Build history of the part. All positions in model axes, mm. A direction names the side the tool comes from. Round coordinates to 2 decimals unless told otherwise and drop trailing zeros. Write each loop counter-clockwise with the first axis right and the second up, starting at its lowest first coordinate (ties: lowest second). Pieces come first, ordered by that corner, then holes.
from build123d import *

# Parameters (mm, degrees)
EXTRUDE_1_DEPTH          = 26.5
SKETCH_3_R               = 1.5
CUT_EXTRUDE_1_DEPTH      = 53.519044165
SKETCH_3_3_R             = 4
CUT_EXTRUDE_2_DEPTH      = 53.519044165
CUT_EXTRUDE_3_DEPTH      = 53.46189093
CUT_EXTRUDE_3_DEPTH_BACK = 53.46189093
SKETCH_4_R               = 1.5
SKETCH_4_R_2             = 5


with BuildPart() as part:
    # Sketch 2 → Extrude 1 (new body)
    with BuildSketch(Plane.XY):
        with BuildLine():
            Line((0, 1), (0, 34))
            Line((0, 34), (3, 34))
            Line((3, 34), (3, 4))
            ThreePointArc((3, 4), (3.292893219, 3.292893219), (4, 3))
            Line((4, 3), (33, 3))
            Line((33, 3), (33, 0))
            Line((33, 0), (1, 0))
            ThreePointArc((1, 0), (0.292893219, 0.292893219), (0, 1))
        make_face()
    extrude(amount=EXTRUDE_1_DEPTH)

    # Sketch 3 → Cut-Extrude 1 (cut, through all)
    with BuildSketch(Plane(origin=(3, 0, 0), x_dir=(0, 0, -1), z_dir=(1, 0, 0))):
        with BuildLine():
            ThreePointArc((-13.25, 34), (-3.880835149, 30.119164851), (0, 20.75))
            Line((0, 20.75), (0, 34))
            Line((0, 34), (-13.25, 34))
        make_face()
        with BuildLine():
            ThreePointArc((-26.5, 20.75), (-22.619164851, 30.119164851), (-13.25, 34))
            Line((-13.25, 34), (-26.5, 34))
            Line((-26.5, 34), (-26.5, 20.75))
        make_face()
        with Locations(Location((-4.75, 20.75, 0), (0, 0, 90))):
            Circle(SKETCH_3_R)
        with Locations(Location((-21.75, 20.75, 0), (0, 0, 90))):
            Circle(SKETCH_3_R)
    extrude(amount=-CUT_EXTRUDE_1_DEPTH, mode=Mode.SUBTRACT)

    # Sketch 3_3 → Cut-Extrude 2 (cut, through all)
    with BuildSketch(Plane(origin=(3, 0, 0), x_dir=(0, 0, -1), z_dir=(1, 0, 0))):
        with Locations(Location((-13.25, 20.75, 0), (0, 0, 90))):
            Circle(SKETCH_3_3_R)
    extrude(amount=-CUT_EXTRUDE_2_DEPTH, mode=Mode.SUBTRACT)

    # Sketch 4 → Cut-Extrude 3 (cut, two sides: drawn at the far end of the back side and taken through both)
    with BuildSketch(Plane(origin=(0, 3, 0), x_dir=(1, 0, 0), z_dir=(0, 1, 0)).offset(-CUT_EXTRUDE_3_DEPTH_BACK)):
        with Locations(Location((10.5, -21.25, 0), (0, 0, 270))):
            Circle(SKETCH_4_R)
        with Locations(Location((10.5, -5.25, 0), (0, 0, 270))):
            Circle(SKETCH_4_R)
        with Locations(Location((26.5, -5.25, 0), (0, 0, 270))):
            Circle(SKETCH_4_R)
        with Locations(Location((18.5, -13.25, 0), (0, 0, 270))):
            Circle(SKETCH_4_R_2)
        with Locations(Location((26.5, -21.25, 0), (0, 0, 270))):
            Circle(SKETCH_4_R)
    extrude(amount=CUT_EXTRUDE_3_DEPTH + CUT_EXTRUDE_3_DEPTH_BACK, mode=Mode.SUBTRACT)


solid = part.part
1) Slice it at D-D (z = 5.25). Write the cut outline in (x, y), plus the area to 3 significant figures.
Results:
outline: (0, 1) arc R1 ccw to (1, 0) - (9, 0) - (9, 3) - (4, 3) arc R1 cw to (3, 4) - (3, 19.34) - (0, 19.34) - close; (0, 22.16) - (3, 22.16) - (3, 31.31) - (0, 31.31) - close; (12, 0) - (25, 0) - (25, 3) - (12, 3) - close; (28, 0) - (33, 0) - (33, 3) - (28, 3) - close
area: 157 mm2
2) Slice it at C-C (y = 23.5). Write the cut outline in (x, z), plus the area to 3 significant figures.
Results:
outline: (0, 0.29) - (3, 0.29) - (3, 10.35) - (0, 10.35) - close; (0, 16.15) - (3, 16.15) - (3, 26.21) - (0, 26.21) - close
area: 60.3 mm2
3) Slice it at B-B (x = 10.5). Write the cut outline in (y, z).
Results:
outline: (0, 0) - (3, 0) - (3, 3.75) - (0, 3.75) - close; (0, 6.75) - (3, 6.75) - (3, 19.75) - (0, 19.75) - close; (0, 22.75) - (3, 22.75) - (3, 26.5) - (0, 26.5) - close
4) Which spindle directions (+Z, -Z, +X, -X, +Y, -Y) get a long thin tool onto all of the face, cutting with end or side? Do faces 1 (the cylindrical face through (27.987, 1.479, 5.055)), 2 (the flat face through (18, 3, 7)). Say none if no direction does.
Results:
face 1: +Y, -Y
face 2: +Z, -Z, +X, +Y
5) Mould opens along X. For faces 3 (the cylindrical face through (1.52, 17.8, 15.95)), 4 (the cylindrical face through (0.301, 0.285, 13.064)), 5 (the cylindrical face through (9.036, 1.479, 4.925)) say: released by +X, released by -X, zero draft, split by the parting line, or undercut.
Results:
face 3: zero draft
face 4: released by -X
face 5: undercut
6) Wall check: L1, parallel to Z at x = 0.9, y = 20.75; L2, parallel to X at y = 2.1, z = 21.25; L3, parallel to Z at x = 1, y = 20. Give the ranges that are in metal, low to high.
Results:
L1: z = 0 to 3.25, 6.25 to 9.25, 17.25 to 20.25, 23.25 to 26.5
L2: x = 0 to 9, 12 to 25, 28 to 33
L3: z = 0 to 3.45, 6.05 to 9.32, 17.18 to 20.45, 23.05 to 26.5
7) Pin check, flat tips, straight feed: pin 1 Ø5 at (x, z) = (26.5, 5.25) entering from +Y; pin 2 Ø1.5 at (y, z) = (29.5, 11.5) entering from +X; pin 3 Ø10 at (x, y) = (6, 27) entering from -Z. Stop position of each tip, or through.
Results:
pin 1: stops at y = 3
pin 2: stops at x = 3
pin 3: stops at z = 0.19
8) Slice it at A-A (x = 18.5). Write the cut outline in (y, z), plus the area to 3 significant figures.
Results:
outline: (0, 0) - (3, 0) - (3, 8.25) - (0, 8.25) - close; (0, 18.25) - (3, 18.25) - (3, 26.5) - (0, 26.5) - close
area: 49.5 mm2
